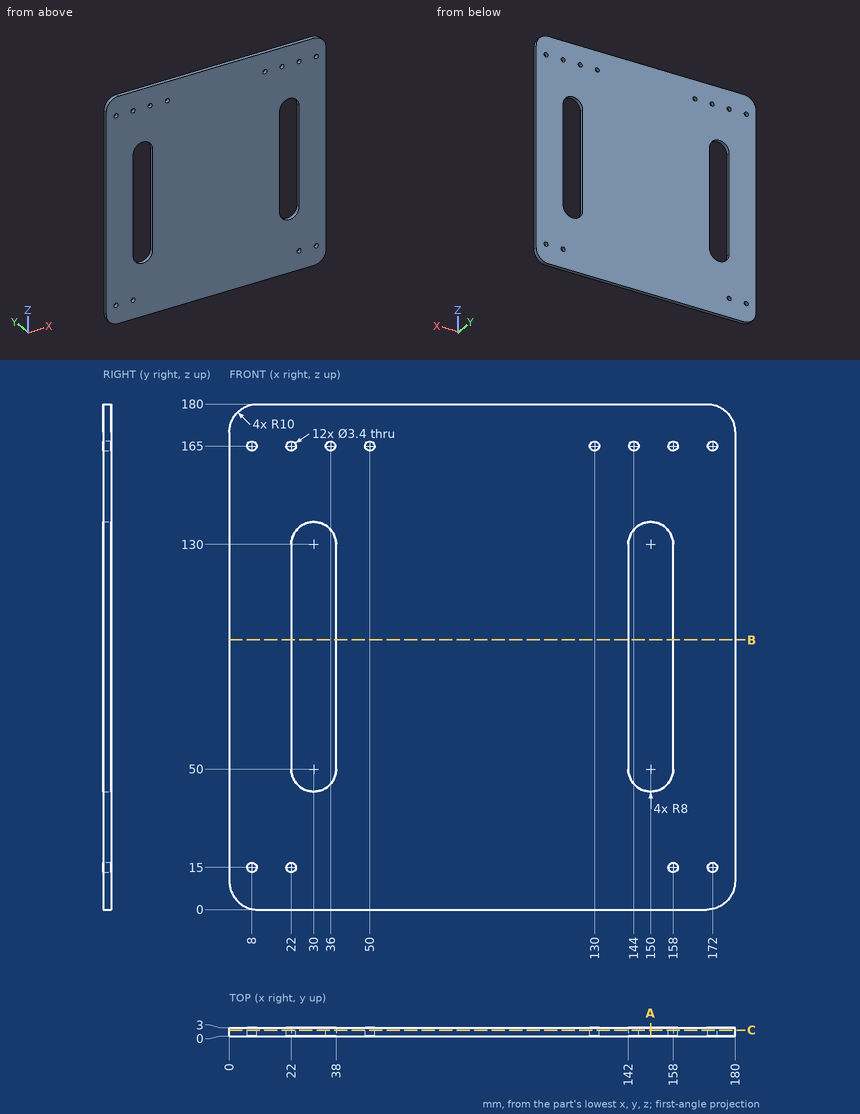
Study the drawing (mm; zero at the part's minimum x, y, z) and answer. Round coordinates to 2 decimals unless told otherwise and drop trailing zeros. Write each loop counter-clockwise with the first axis right and the second up, starting at its lowest first coordinate (ties: lowest second). Pieces come first, ordered by that corner, then holes.
1) Consider probe 1 along X at (y, z) = (1.75, 15); probe 2 along X at (y, z) = (1.5, 116); probe 3 along Z at (x, y) = (130, 1.2). Determine where each line is inside the solid, lowest interval first.
2) A cutting plane is placed at C-C on y = 2.1. Give the number of separate pieces and of enclosed holes in the cut face, and give its area (3 significant figures).
3) A cutting plane is placed at B-B on z = 96. Determine the outline of the cut face in (x, y), and give its area (3 significant figures).
4) A cutting plane is placed at A-A on x = 150. Determine the outline of the cut face in (y, z), and give its area (3 significant figures).
Entries:
1. probe 1: x = 0 to 6.3, 9.7 to 20.3, 23.7 to 156.3, 159.7 to 170.3, 173.7 to 180
1. probe 2: x = 0 to 22, 38 to 142, 158 to 180
1. probe 3: z = 0 to 163.3, 166.7 to 180
2. separate pieces: 1
2. enclosed holes: 14
2. area: 29,200 mm2
3. outline: (0, 0) - (22, 0) - (22, 3) - (0, 3) - close; (38, 0) - (142, 0) - (142, 3) - (38, 3) - close; (158, 0) - (180, 0) - (180, 3) - (158, 3) - close
3. area: 444 mm2
4. outline: (0, 0) - (3, 0) - (3, 42) - (0, 42) - close; (0, 138) - (3, 138) - (3, 180) - (0, 180) - close
4. area: 252 mm2
